The figure shows three views and two pictorial views of one solid part (mm, origin at its lowest corner). Answer the questions. Give positions to 0.01 mm unless a question says otherwise; leave off trailing zeros. Loops run counter-clockwise (first coordinate to the right, second up) from the corner with the lowest first, then second, coordinate; pieces in that order, holes last. Notation, with made-up numbers: M -25,9 L 17,9 A32 cw 17,45 Z; hole C -16.5,-3 d8. An arc over 180 degrees is marked long. Answer in a Markdown table with one row per item. Add a question column.
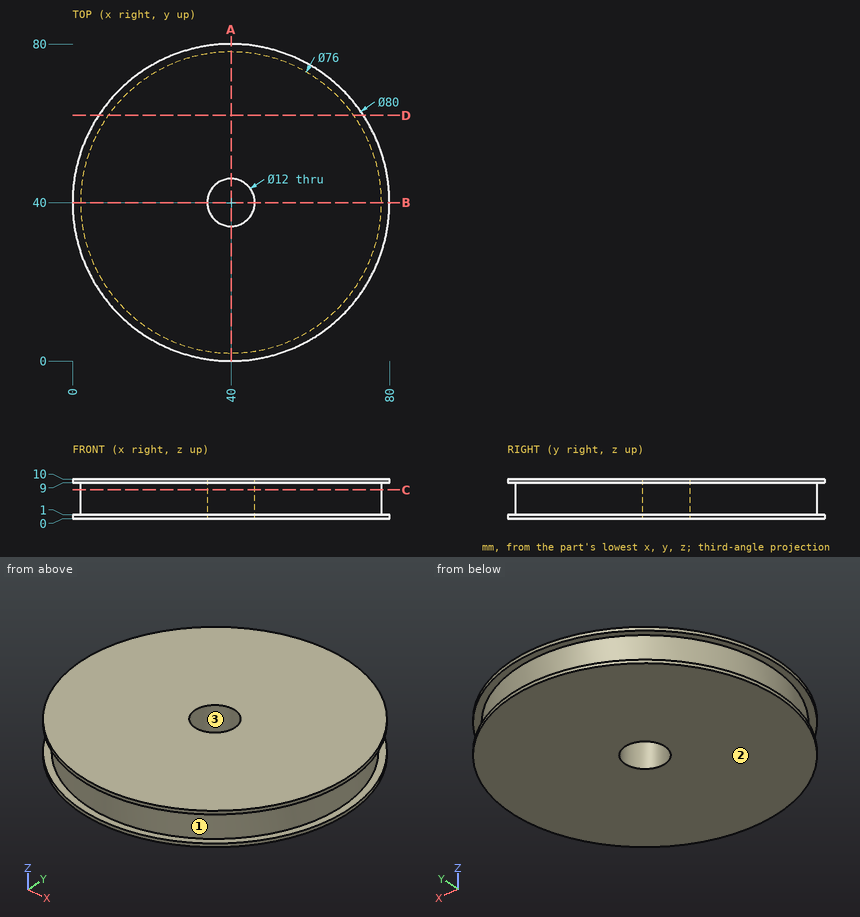
(1) Section D-D, the plane y = 62 is taken. Determine the outline of the cut face in (x, z).
(2) Consider line 1 along Y through (x, z) = (40, 4.75); line 2 along X through (y, z) = (45.5, 2.25); line 3 along Y through (x, z) = (43.5, 1.5). Determine where each line is inside the solid, lowest interval first. Write a range as from..to.
(3) Section C-C, the plane z = 7.25 is taken. Determine the outline of the cut face in (x, y), and give its area (3 significant figures).
(4) Section A-A, the plane x = 40 is taken. Determine the outline of the cut face in (y, z).
(5) The mould has two halves that part along X. Classify the marked faces 1, 2 and 3: pulls with the +X half, pulls with the -X half, needs draft (parallel to the pull), parting line crosses it, or undercut.
(6) Each of these flat-tipped pins is pushed along its axis until it touches: P1, Ø5, axis at x = 45.5, z = 6, coming from the -Y side; P2, Ø1.5, axis at x = 34.5, z = 1.5, coming from the -Y side; P3, Ø6, axis at x = 52, z = 5, coming from the -Y side; P4, Ø7, axis at x = 40, y = 40, coming from the -Z side. Where does it stop, or does it pass through?
Numbers:
| question | item | result |
|---|---|---|
| 1 | outline | M 6.59,0 L 73.41,0 L 73.41,1 L 70.98,1 L 70.98,9 L 73.41,9 L 73.41,10 L 6.59,10 L 6.59,9 L 9.02,9 L 9.02,1 L 6.59,1 Z |
| 2 | line 1 | y = 2..34, 46..78 |
| 2 | line 2 | x = 2.4..37.6, 42.4..77.6 |
| 2 | line 3 | y = 2.16..35.13, 44.87..77.84 |
| 3 | outline | C 40,40 d76; hole C 40,40 d12 |
| 3 | area | 4,420 mm² |
| 4 | outline | M 0,0 L 34,0 L 34,10 L 0,10 L 0,9 L 2,9 L 2,1 L 0,1 Z; M 46,0 L 80,0 L 80,1 L 78,1 L 78,9 L 80,9 L 80,10 L 46,10 Z |
| 5 | face 1 | parting line crosses it |
| 5 | face 2 | needs draft |
| 5 | face 3 | undercut |
| 6 | P1 | stops at y = 2.12 |
| 6 | P2 | stops at y = 0.31 |
| 6 | P3 | stops at y = 3.08 |
| 6 | P4 | passes through |
